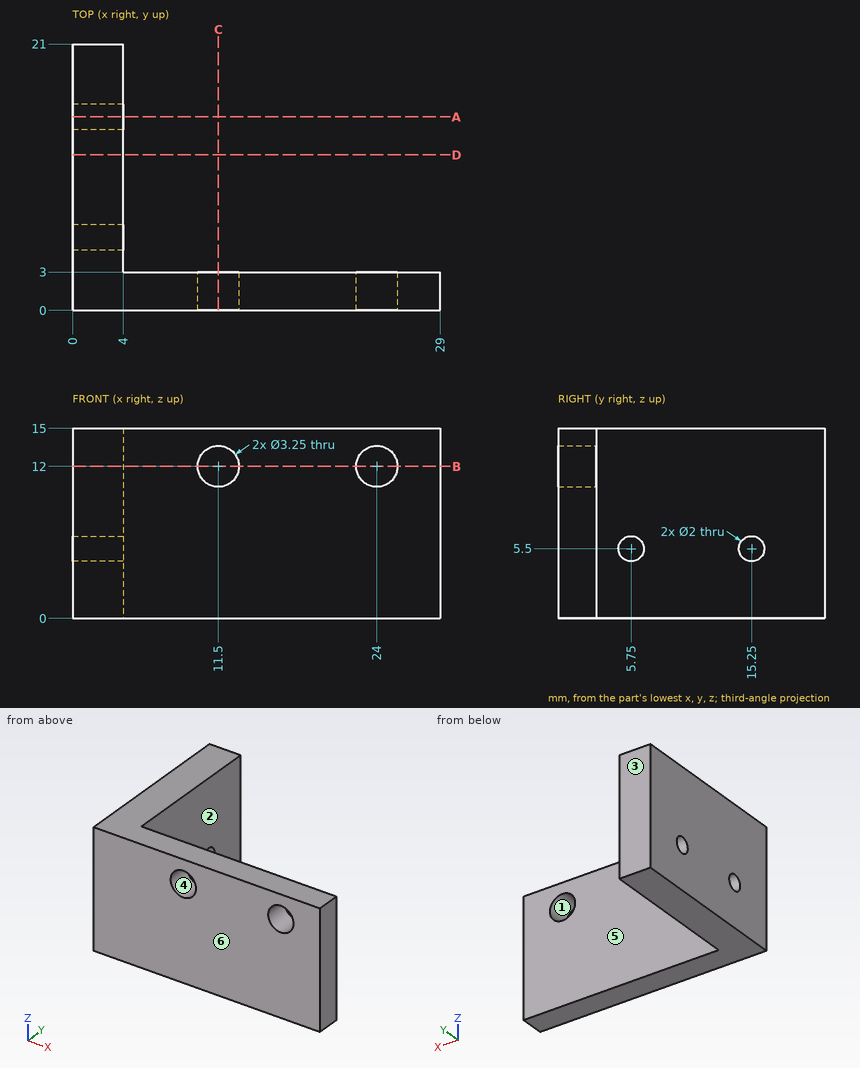
Drawing for the job (mm, zero at the part's lowest x, y, z). A direction names the side the tool comes from. Give positions to 0.01 mm unless a question says otherwise; leave off trailing zeros. Write each loop counter-clockwise with the first axis right and the second up, starting at its lowest first coordinate (ties: lowest second). Pieces come first, ordered by that corner, then holes. Notation, with made-up numbers: (29, 40.25) - (47, 40.25) arc R8 ccw to (47, 47.25) - close; hole circle Ø1 at (-13.5, 61.5). An arc over 180 degrees is marked (long way). Answer as CSV lines item,"result".
Q1. 3-axis set-ups, long thin cutter, end or side, ignore diameter. For the marked faces 5 and 6: which of +Z, -Z, +X, -X, +Y, -Y reach the whole face in a straight line?
Result set:
face 5,"+Z, -Z, +X, +Y"
face 6,"+Z, -Z, +X, -X, -Y"
Q2. Band-saw the part on B-B (z = 12). Give the cut face in (x, y) (3 decimals), and give its area (4 significant figures).
Result set:
outline,"(0, 0) - (9.875, 0) - (9.875, 3) - (4, 3) - (4, 21) - (0, 21) - close; (13.125, 0) - (22.375, 0) - (22.375, 3) - (13.125, 3) - close; (25.625, 0) - (29, 0) - (29, 3) - (25.625, 3) - close"
area,"139.5 mm²"
Q3. Flat gauge pins, fed straight in: pin 1 Ø4.5 at (x, z) = (20, 9) entering from +Y; pin 2 Ø3 at (y, z) = (7, 3.5) entering from +X. Where does each tip first touch, or does it go through?
Result set:
pin 1,"y = 3"
pin 2,"x = 4"
Q4. Band-saw the part on D-D (y = 12.25). Give the cut face in (x, z).
Result set:
outline,"(0, 0) - (4, 0) - (4, 15) - (0, 15) - close"
Q5. Band-saw the part on A-A (y = 15.25). Give the cut face in (x, z).
Result set:
outline,"(0, 0) - (4, 0) - (4, 4.5) - (0, 4.5) - close; (0, 6.5) - (4, 6.5) - (4, 15) - (0, 15) - close"
Q6. Drill centre lines: line 1 (Y direction, x = 1.7, z = 5.5); line 2 (X direction, y = 1.55, z = 12) (3 decimals); line 3 (Z direction, x = 11.5, y = 1.5) (3 decimals). Where is each one in solid material? Low to high. Write a range as from..to.
Result set:
line 1,"0..4.75, 6.75..14.25, 16.25..21"
line 2,"0..9.875, 13.125..22.375, 25.625..29"
line 3,"0..10.375, 13.625..15"
Q7. Band-saw the part on C-C (x = 11.5). Give the cut face in (y, z) (3 decimals), and give its area (4 significant figures).
Result set:
outline,"(0, 0) - (3, 0) - (3, 10.375) - (0, 10.375) - close; (0, 13.625) - (3, 13.625) - (3, 15) - (0, 15) - close"
area,"35.25 mm²"
Q8. Pull direction X, two halves, no side cores. Call the marked faces 1, 2, 3 and 4: released by +X, released by -X, zero draft, split by the parting line, or undercut.
Result set:
face 1,"undercut"
face 2,"released by +X"
face 3,"zero draft"
face 4,"undercut"
